For this review, take the finished solid that the model builds, in its own axes (mm). Give positions to 0.01 mm unless a question says otherwise; leave off trailing zeros. Write each loop counter-clockwise with the first axis right and the second up, starting at its lowest first coordinate (ties: lowest second). Pieces come first, ordered by that corner, then holes. Notation, with made-up numbers: (38, -38.75) -> (73, -38.75) arc R3 cw to (73, -34.75) -> close; hole circle Ø9 at (13.5, 83). An arc over 180 degrees is marked (long way). Return JSON: item names as keys, results as strings.
from build123d import *

# Parameters (mm, degrees)
ESQUISSE1_R        = 1.65
ESQUISSE1_R_2      = 7.5
ESQUISSE1_R_3      = 12.5
ESQUISSE1_W        = 5.4
ESQUISSE1_H        = 50.4
BOSS_EXTRU_1_DEPTH = 5


with BuildPart() as part:
    # Esquisse1 → Boss.-Extru.1 (new body)
    with BuildSketch(Plane.XY):
        with BuildLine():
            Line((-220, 100), (-0.145812859, 100))
            Line((-0.145812859, 100), (9.854187141, 100))
            Line((9.854187141, 100), (220, 100))
            Line((220, 100), (220, -100))
            Line((220, -100), (47.761564371, -100))
            Line((47.761564371, -100), (47.761564371, -18.538015518))
            Line((47.761564371, -18.538015518), (46.481557411, -18.538015518))
            Line((46.481557411, -18.538015518), (46.481557411, -17.125104692))
            ThreePointArc((46.481557411, -17.125104692), (45, -8.375988591), (43.518442589, -17.125104692))
            Line((43.518442589, -17.125104692), (43.518442589, -18.538015518))
            Line((43.518442589, -18.538015518), (31.481557411, -18.538015518))
            Line((31.481557411, -18.538015518), (31.481557411, -17.125104692))
            ThreePointArc((31.481557411, -17.125104692), (30, -8.375988591), (28.518442589, -17.125104692))
            Line((28.518442589, -17.125104692), (28.518442589, -18.538015518))
            Line((28.518442589, -18.538015518), (16.481557411, -18.538015518))
            Line((16.481557411, -18.538015518), (16.481557411, -17.125104692))
            ThreePointArc((16.481557411, -17.125104692), (15, -8.375988591), (13.518442589, -17.125104692))
            Line((13.518442589, -17.125104692), (13.518442589, -18.538015518))
            Line((13.518442589, -18.538015518), (1.481557411, -18.538015518))
            Line((1.481557411, -18.538015518), (1.481557411, -17.125104692))
            ThreePointArc((1.481557411, -17.125104692), (0, -8.375988591), (-1.481557411, -17.125104692))
            Line((-1.481557411, -17.125104692), (-1.481557411, -18.538015518))
            Line((-1.481557411, -18.538015518), (-13.518442589, -18.538015518))
            Line((-13.518442589, -18.538015518), (-13.518442589, -17.125104692))
            ThreePointArc((-13.518442589, -17.125104692), (-15, -8.375988591), (-16.481557411, -17.125104692))
            Line((-16.481557411, -17.125104692), (-16.481557411, -18.538015518))
            Line((-16.481557411, -18.538015518), (-28.518442589, -18.538015518))
            Line((-28.518442589, -18.538015518), (-28.518442589, -17.125104692))
            ThreePointArc((-28.518442589, -17.125104692), (-30, -8.375988591), (-31.481557411, -17.125104692))
            Line((-31.481557411, -17.125104692), (-31.481557411, -18.538015518))
            Line((-31.481557411, -18.538015518), (-43.518442589, -18.538015518))
            Line((-43.518442589, -18.538015518), (-43.518442589, -17.125104692))
            ThreePointArc((-43.518442589, -17.125104692), (-45, -8.375988591), (-46.481557411, -17.125104692))
            Line((-46.481557411, -17.125104692), (-46.481557411, -18.538015518))
            Line((-46.481557411, -18.538015518), (-47.761564371, -18.538015518))
            Line((-47.761564371, -18.538015518), (-47.761564371, -100))
            Line((-47.761564371, -100), (-220, -100))
            Line((-220, -100), (-220, 100))
        make_face()
        with Locations((-152.3, -94.376990981)):
            Circle(ESQUISSE1_R, mode=Mode.SUBTRACT)
        with Locations((-67.3, -94.376990981)):
            Circle(ESQUISSE1_R, mode=Mode.SUBTRACT)
        with Locations(Location((67.3, -94.376990981, 0), (0, 0, 180))):
            Circle(ESQUISSE1_R, mode=Mode.SUBTRACT)
        with Locations(Location((152.3, -94.376990981, 0), (0, 0, 180))):
            Circle(ESQUISSE1_R, mode=Mode.SUBTRACT)
        with Locations((-194.730758968, 77.3)):
            Circle(ESQUISSE1_R_2, mode=Mode.SUBTRACT)
        with Locations((-194.730758968, -10.2)):
            Circle(ESQUISSE1_R_2, mode=Mode.SUBTRACT)
        with Locations((-194.730758968, 29.8)):
            Circle(ESQUISSE1_R_2, mode=Mode.SUBTRACT)
        with Locations(Location((194.730758968, -10.2, 0), (0, 0, 180))):
            Circle(ESQUISSE1_R_2, mode=Mode.SUBTRACT)
        with Locations(Location((194.730758968, 77.3, 0), (0, 0, 180))):
            Circle(ESQUISSE1_R_2, mode=Mode.SUBTRACT)
        with Locations(Location((194.730758968, 29.8, 0), (0, 0, 180))):
            Circle(ESQUISSE1_R_2, mode=Mode.SUBTRACT)
        with Locations((110.068688128, 14.7)):
            Circle(ESQUISSE1_R_3, mode=Mode.SUBTRACT)
        with Locations((0, 14.7)):
            Circle(ESQUISSE1_R_3, mode=Mode.SUBTRACT)
        with Locations(Location((-110.068688128, 14.7, 0), (0, 0, 180))):
            Circle(ESQUISSE1_R_3, mode=Mode.SUBTRACT)
        with Locations((110.068688128, -25.3)):
            Circle(ESQUISSE1_R_3, mode=Mode.SUBTRACT)
        with Locations(Location((-110.068688128, -25.3, 0), (0, 0, 180))):
            Circle(ESQUISSE1_R_3, mode=Mode.SUBTRACT)
        with Locations((110.068688128, -65.3)):
            Circle(ESQUISSE1_R_3, mode=Mode.SUBTRACT)
        with Locations(Location((-110.068688128, -65.3, 0), (0, 0, 180))):
            Circle(ESQUISSE1_R_3, mode=Mode.SUBTRACT)
        Polygon((-70, 89.8), (-70, -60.4), (-64.6, -60.4), (-64.6, 89.8), (-24.6, 89.8), (-24.6, 95), (-75, 95), (-75, 89.8), align=None, mode=Mode.SUBTRACT)
        Polygon((-155, 89.8), (-155, -60.4), (-149.6, -60.4), (-149.6, 89.8), (-124.6, 89.8), (-124.6, 95), (-175, 95), (-175, 89.8), align=None, mode=Mode.SUBTRACT)
        Polygon((155, -60.4), (149.6, -60.4), (149.6, 89.8), (125, 89.8), (125, 95), (175.4, 95), (175.4, 89.8), (155, 89.8), align=None, mode=Mode.SUBTRACT)
        Polygon((64.6, 89.8), (64.6, -60.4), (70, -60.4), (70, 89.8), (75.4, 89.8), (75.4, 95), (25, 95), (25, 89.8), align=None, mode=Mode.SUBTRACT)
        with Locations((212.3, -50.2)):
            Rectangle(ESQUISSE1_W, ESQUISSE1_H, mode=Mode.SUBTRACT)
        with Locations((212.3, 29.8)):
            Rectangle(ESQUISSE1_W, ESQUISSE1_H, mode=Mode.SUBTRACT)
        with Locations((-212.3, -50.2)):
            Rectangle(ESQUISSE1_W, ESQUISSE1_H, mode=Mode.SUBTRACT)
        with Locations((-212.3, 29.8)):
            Rectangle(ESQUISSE1_W, ESQUISSE1_H, mode=Mode.SUBTRACT)
    extrude(amount=BOSS_EXTRU_1_DEPTH)


solid = part.part
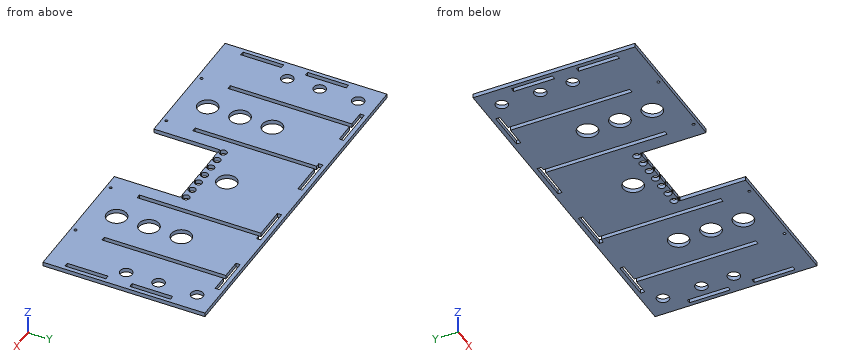
1. Add section C-C, the plane y = -65.3. State the section outline as (x, z) points, plus the area to 3 significant figures.
Results found:
{"outline": "(-220, 0) -> (-215, 0) -> (-215, 5) -> (-220, 5) -> close; (-209.6, 0) -> (-122.57, 0) -> (-122.57, 5) -> (-209.6, 5) -> close; (-97.57, 0) -> (-47.76, 0) -> (-47.76, 5) -> (-97.57, 5) -> close; (47.76, 0) -> (97.57, 0) -> (97.57, 5) -> (47.76, 5) -> close; (122.57, 0) -> (209.6, 0) -> (209.6, 5) -> (122.57, 5) -> close; (215, 0) -> (220, 0) -> (220, 5) -> (215, 5) -> close", "area": "1,420 mm²"}
2. Add section B-B, the plane y = 77.3. State the section outline as (x, z) points.
Results found:
{"outline": "(-220, 0) -> (-202.23, 0) -> (-202.23, 5) -> (-220, 5) -> close; (-187.23, 0) -> (-155, 0) -> (-155, 5) -> (-187.23, 5) -> close; (-149.6, 0) -> (-70, 0) -> (-70, 5) -> (-149.6, 5) -> close; (-64.6, 0) -> (64.6, 0) -> (64.6, 5) -> (-64.6, 5) -> close; (70, 0) -> (149.6, 0) -> (149.6, 5) -> (70, 5) -> close; (155, 0) -> (187.23, 0) -> (187.23, 5) -> (155, 5) -> close; (202.23, 0) -> (220, 0) -> (220, 5) -> (202.23, 5) -> close"}
3. To check wall thickness, follow probe 1 along X at (y, z) = (63, 3.15); probe 2 along X at (y, z) = (-83, 2.6); probe 3 along X at (y, z) = (-74, 4.75). State the ranges of each line that lie inside material, in increasing order.
Results found:
{"probe 1": "x = -220 to -155, -149.6 to -70, -64.6 to 64.6, 70 to 149.6, 155 to 220", "probe 2": "x = -220 to -47.76, 47.76 to 220", "probe 3": "x = -220 to -215, -209.6 to -119.04, -101.09 to -47.76, 47.76 to 101.09, 119.04 to 209.6, 215 to 220"}
4. Add section D-D, the plane y = 14.7. Count the separate pieces of the cut face and the enclosed holes in it, plus the area to 3 significant figures.
Results found:
{"separate pieces": "10", "enclosed holes": "0", "area": "1,660 mm²"}
5. Add section A-A, the plane x = 55. State the section outline as (y, z) points, plus the area to 3 significant figures.
Results found:
{"outline": "(-100, 0) -> (89.8, 0) -> (89.8, 5) -> (-100, 5) -> close; (95, 0) -> (100, 0) -> (100, 5) -> (95, 5) -> close", "area": "974 mm²"}
